Source: CAD feature listing. Evaluate the final solid. Frame: model axes, mm. Face numbers are marked on the shaded views. A direction names the side the tool comes from. Coordinates: 2 decimals unless noted, no trailing zeros. Write each loop counter-clockwise with the first axis right and the second up, starting at its lowest first coordinate (ties: lowest second). Pieces come first, ordered by that corner, then holes. Notation, with made-up numbers: (30, 72.25) - (59, 72.25) arc R29 ccw to (59, 93.25) - close; hole circle Ø1 at (85, -13.75). An arc over 180 degrees is marked (long way). One line per item, written item: value.
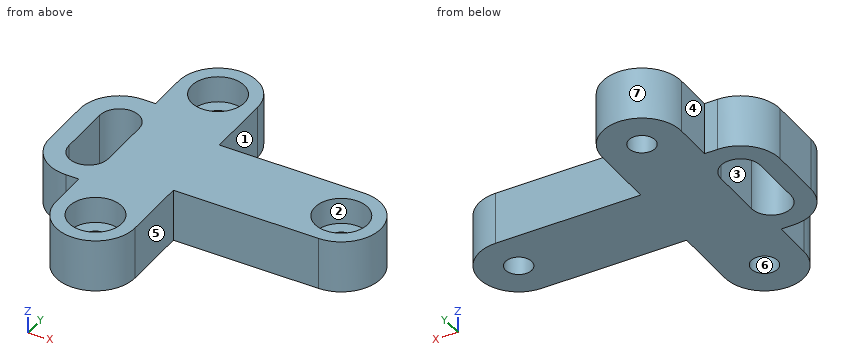
from build123d import *

# Parameters (mm, degrees)
IZIM1_R                     = 10
Y_KSEKLIK_EKSTR_ZYON1_DEPTH = 20
IZIM1_3_R                   = 10
IZIM1_3_R_2                 = 5
Y_KSEKLIK_EKSTR_ZYON2_DEPTH = 10


with BuildPart() as part:
    # izim1 → Y_kseklik-Ekstr_zyon1 (new body)
    with BuildSketch(Plane.XY):
        with BuildLine():
            Line((15.000607379, -15), (70.000607379, -15))
            ThreePointArc((70.000607379, -15), (85.000607379, 0), (70.000607379, 15))
            Line((70.000607379, 15), (15.000607379, 15))
            Line((15.000607379, 15), (15.000607379, 40))
            ThreePointArc((15.000607379, 40), (0.000607379, 55), (-14.999392621, 40))
            Line((-14.999392621, 40), (-14.999392621, 25))
            Line((-14.999392621, 25), (-20, 25))
            ThreePointArc((-20, 25), (-30.606601718, 20.606601718), (-35, 10))
            Line((-35, 10), (-35, -10))
            ThreePointArc((-35, -10), (-30.606601718, -20.606601718), (-20, -25))
            Line((-20, -25), (-14.999392621, -25))
            Line((-14.999392621, -25), (-14.999392621, -40))
            ThreePointArc((-14.999392621, -40), (0.000607379, -55), (15.000607379, -40))
            Line((15.000607379, -40), (15.000607379, -15))
        make_face()
        with Locations((0.000607379, -40)):
            Circle(IZIM1_R, mode=Mode.SUBTRACT)
        with Locations((0.000607379, 40)):
            Circle(IZIM1_R, mode=Mode.SUBTRACT)
        with Locations((70.000607379, 0)):
            Circle(IZIM1_R, mode=Mode.SUBTRACT)
        with BuildLine():
            ThreePointArc((-27.5, -10), (-20, -17.5), (-12.5, -10))
            Line((-12.5, -10), (-12.5, 10))
            ThreePointArc((-12.5, 10), (-20, 17.5), (-27.5, 10))
            Line((-27.5, 10), (-27.5, -10))
        make_face(mode=Mode.SUBTRACT)
    extrude(amount=Y_KSEKLIK_EKSTR_ZYON1_DEPTH)

    # izim1_3 → Y_kseklik-Ekstr_zyon2 (add)
    # profile 1 of 3: a face of its own
    with BuildSketch(Plane.XY):
        with Locations((0.000607379, 40)):
            Circle(IZIM1_3_R)
        with Locations((0.000607379, 40)):
            Circle(IZIM1_3_R_2, mode=Mode.SUBTRACT)
    # profile 2 of 3: a face of its own
    with BuildSketch(Plane.XY):
        with Locations((0.000607379, -40)):
            Circle(IZIM1_3_R)
        with Locations((0.000607379, -40)):
            Circle(IZIM1_3_R_2, mode=Mode.SUBTRACT)
    # profile 3 of 3: a face of its own
    with BuildSketch(Plane.XY):
        with Locations((70.000607379, 0)):
            Circle(IZIM1_3_R)
        with Locations((70.000607379, 0)):
            Circle(IZIM1_3_R_2, mode=Mode.SUBTRACT)
    extrude(amount=Y_KSEKLIK_EKSTR_ZYON2_DEPTH)


solid = part.part
1) Material intervals for line 1 (Y direction, x = 8, z = 13); line 2 (Y direction, x = 8.5, z = 15.25); line 3 (Y direction, x = 51, z = 4), sorted ascending.
Values found:
line 1: -52.69 to -46, -34 to 34, 46 to 52.69
line 2: -52.36 to -45.27, -34.73 to 34.73, 45.27 to 52.36
line 3: -15 to 15
2) Reachability of the marked faces 1, 2, 3 and 4 from +Z, -Z, +X, -X, +Y, -Y: full face, straight path, thin tool, end or side. Return the list, or none.
Values found:
face 1: +Z, -Z, +X, +Y
face 2: +Z
face 3: +Z, -Z
face 4: +Z, -Z, -X, +Y
3) Contact query for flat-ended pins moving along their axis: P1, Ø6, axis at x = 0, y = -40, coming from the +Z side; P2, Ø12, axis at y = 34.5, z = 17, coming from the +X side; P3, Ø12, axis at x = 52.5, z = 16.5, coming from the +Y side; P4, Ø1.5, axis at y = 5.5, z = 7.5, coming from the +X side. Output: stop coordinate, or through.
Values found:
P1: through
P2: x = 15
P3: y = 15
P4: x = 84.23
4) Draft query along X for the marked faces 5, 6 and 7. Return one class per face: released by +X, released by -X, zero draft, split by the parting line, or undercut.
Values found:
face 5: released by +X
face 6: undercut
face 7: split by the parting line
5) Section query A-A on y = 0. Output: boundary loops of the cut face in (x, z).
Values found:
outline: (-35, 0) - (-27.5, 0) - (-27.5, 20) - (-35, 20) - close; (-12.5, 0) - (65, 0) - (65, 10) - (60, 10) - (60, 20) - (-12.5, 20) - close; (75, 0) - (85, 0) - (85, 20) - (80, 20) - (80, 10) - (75, 10) - close
6) Section query B-B on x = -22. Output: boundary loops of the cut face in (y, z).
Values found:
outline: (-24.87, 0) - (-17.23, 0) - (-17.23, 20) - (-24.87, 20) - close; (17.23, 0) - (24.87, 0) - (24.87, 20) - (17.23, 20) - close
7) Section query D-D on y = -33. Output: boundary loops of the cut face in (x, z), then the cut area to 3 significant figures.
Values found:
outline: (-15, 0) - (15, 0) - (15, 20) - (7.14, 20) - (7.14, 10) - (-7.14, 10) - (-7.14, 20) - (-15, 20) - close
area: 457 mm2
8) Section query C-C on z = 13.5. Output: boundary loops of the cut face in (x, y).
Values found:
outline: (-35, -10) arc R15 ccw to (-20, -25) - (-15, -25) - (-15, -40) arc R15 ccw to (15, -40) - (15, -15) - (70, -15) arc R15 ccw to (70, 15) - (15, 15) - (15, 40) arc R15 ccw to (-15, 40) - (-15, 25) - (-20, 25) arc R15 ccw to (-35, 10) - close; hole (-27.5, -10) arc R7.5 ccw to (-12.5, -10) - (-12.5, 10) arc R7.5 ccw to (-27.5, 10) - close; hole circle Ø20 at (0, -40); hole circle Ø20 at (0, 40); hole circle Ø20 at (70, 0)
